Part model, mm, in its own coordinate system. Face numbers are marked on the shaded views. A direction names the side the tool comes from. Round coordinates to 2 decimals unless told otherwise and drop trailing zeros. Loops run counter-clockwise (first coordinate to the right, second up) from the corner with the lowest first, then second, coordinate; pieces in that order, holes last.
from build123d import *

# Parameters (mm, degrees)
F1_DEPTH = 60
F2_W     = 480.000014
F2_H     = 330.000014
F3_DEPTH = 55


with BuildPart() as f1:
    # F0 (on Top) → F1 (new body)
    with BuildSketch(Plane.XY):
        with BuildLine():
            ThreePointArc((250, 165), (247.071068, 172.071068), (240, 175))
            Line((240, 175), (-240, 175))
            ThreePointArc((-240, 175), (-247.071068, 172.071068), (-250, 165))
            Line((-250, 165), (-250, -165))
            ThreePointArc((-250, -165), (-247.071068, -172.071068), (-240, -175))
            Line((-240, -175), (240, -175))
            ThreePointArc((240, -175), (247.071068, -172.071068), (250, -165))
            Line((250, -165), (250, 165))
        make_face()
    extrude(amount=F1_DEPTH)

    # F2 (on face) → F3 (cut)
    with BuildSketch(Plane.XY):
        Rectangle(F2_W, F2_H)
    extrude(amount=F3_DEPTH, mode=Mode.SUBTRACT)


solid = f1.part
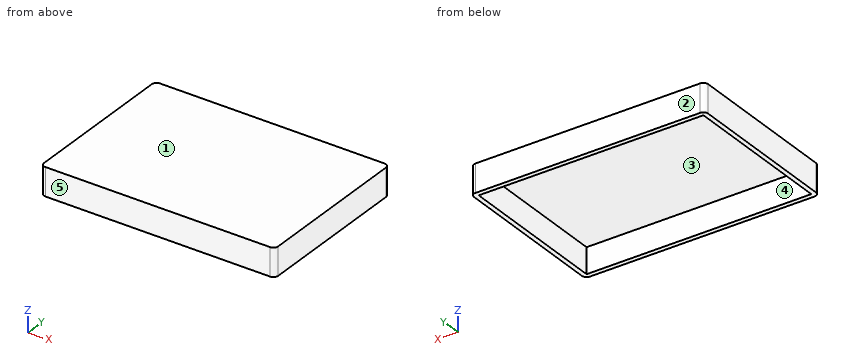
1) Slice it at A-A, the plane z = 24. Give the cut face in (x, y).
Values:
outline: (-250, -165) arc R10 ccw to (-240, -175) - (240, -175) arc R10 ccw to (250, -165) - (250, 165) arc R10 ccw to (240, 175) - (-240, 175) arc R10 ccw to (-250, 165) - close; hole (-240, -165) - (240, -165) - (240, 165) - (-240, 165) - close
2) Tool access for the marked faces 4 and 5: list every direction of +Z, -Z, +X, -X, +Y, -Y with a clear straight run to the whole face (end or side of a thin tool).
Values:
face 4: -Z
face 5: +Z, -Z, +X, -X, -Y
3) Slice it at B-B, the plane x = 5. Give the cut face in (y, z).
Values:
outline: (-175, 0) - (-165, 0) - (-165, 55) - (165, 55) - (165, 0) - (175, 0) - (175, 60) - (-175, 60) - close
4) Slice it at C-C, the plane y = -41. Give the cut face in (x, z), then the cut area to 3 significant figures.
Values:
outline: (-250, 0) - (-240, 0) - (-240, 55) - (240, 55) - (240, 0) - (250, 0) - (250, 60) - (-250, 60) - close
area: 3,600 mm2
5) Wall check: line 1 along Y through (x, z) = (-17.5, 4.5); line 2 along X through (y, z) = (138, 49); line 3 along Z through (x, y) = (202.5, -106). Give the ranges that are in metal, low to high.
Values:
line 1: y = -175 to -165, 165 to 175
line 2: x = -250 to -240, 240 to 250
line 3: z = 55 to 60
6) Mould opens along Y. For the marked faces 1, 2 and 3 say: released by +Y, released by -Y, zero draft, split by the parting line, or undercut.
Values:
face 1: zero draft
face 2: released by +Y
face 3: undercut
